Geometry check sheet. Reference: the model listing, model coordinates, mm. A direction names the side the tool comes from. Round coordinates to 2 decimals unless told otherwise and drop trailing zeros. Order: outer loops, then holes, each group sorted by start corner. A loop starts at its lowest first (then second) coordinate and runs counter-clockwise, first axis right, second up. Notation, with made-up numbers: (13.25, 15) -> (26.25, 15) arc R19 ccw to (26.25, 36) -> close; hole circle Ø5 at (51.5, -24). An arc over 180 degrees is marked (long way). Answer as a JSON object with one key per item and string values. Group by question number.
from build123d import *

# Parameters (mm, degrees)
SKETCH2_R           = 2.25
BOSS_EXTRUDE1_DEPTH = 6.35


with BuildPart() as part:
    # Sketch2 → Boss-Extrude1 (new body)
    with BuildSketch(Plane(origin=(0, 0, 71.255), x_dir=(-1, 0, 0), z_dir=(0, 0, -1))):
        with BuildLine():
            Line((-39.5, -8), (39.5, -8))
            ThreePointArc((39.5, -8), (43.035533906, -9.464466094), (44.5, -13))
            Line((44.5, -13), (44.5, -12.496398734))
            ThreePointArc((44.5, -12.496398734), (51.25, -19.246398734), (58, -12.496398734))
            Line((58, -12.496398734), (58, 23.184046239))
            ThreePointArc((58, 23.184046239), (51.25, 29.934046239), (44.5, 23.184046239))
            Line((44.5, 23.184046239), (44.5, 13))
            ThreePointArc((44.5, 13), (43.035533906, 9.464466094), (39.5, 8))
            Line((39.5, 8), (-39.5, 8))
            ThreePointArc((-39.5, 8), (-43.035533906, 9.464466094), (-44.5, 13))
            Line((-44.5, 13), (-44.5, 23.184046239))
            ThreePointArc((-44.5, 23.184046239), (-51.25, 29.934046239), (-58, 23.184046239))
            Line((-58, 23.184046239), (-58, -12.496398734))
            ThreePointArc((-58, -12.496398734), (-51.539037503, -19.240207548), (-44.524753386, -13.073943522))
            Line((-44.524753386, -13.073943522), (-44.481664158, -12.572189046))
            ThreePointArc((-44.481664158, -12.572189046), (-42.880898196, -9.316316058), (-39.5, -8))
        make_face()
        with Locations((47.5, 0)):
            Circle(SKETCH2_R, mode=Mode.SUBTRACT)
        with Locations((-47.5, 0)):
            Circle(SKETCH2_R, mode=Mode.SUBTRACT)
        with Locations((51.25, 23.184046239)):
            Circle(SKETCH2_R, mode=Mode.SUBTRACT)
        with Locations((51.25, -12.496398734)):
            Circle(SKETCH2_R, mode=Mode.SUBTRACT)
        with Locations((-51.25, -12.496398734)):
            Circle(SKETCH2_R, mode=Mode.SUBTRACT)
        with Locations((-51.25, 23.184046239)):
            Circle(SKETCH2_R, mode=Mode.SUBTRACT)
    extrude(amount=BOSS_EXTRUDE1_DEPTH)


solid = part.part
Item 1: Sectioned sample at D-D, the plane x = 51.25. Enter the section's corners in (y, z) (3 decimals), then the cut area to 3 significant figures.
Item 2: Sectioned sample at A-A, the plane y = 0. Enter the section's corners in (x, z) (3 decimals), then the cut area to 3 significant figures.
Item 3: Mould release check, pull along X, two halves, no side actions. Record for faces 1 (the cylindrical face through (53.498, -12.397, 68.124)), 2 (the cylindrical face through (53.498, 23.283, 68.124)), 3 (the flat face through (58, 6, 68)), 4 (the flat face through (1, 0, 64.905)): pulls with the +X half, pulls with the -X half, needs draft (parallel to the pull), parting line crosses it, or undercut.
Item 4: Thickness scan on L1, parallel to Y at x = -51, z = 66.25; L2, parallel to X at y = 18, z = 68; L3, parallel to X at y = 23.5, z = 65.5. Record the ranges inside material, lowest first.
Item 5: Sectioned sample at B-B, the plane y = 19. Enter the section's corners in (x, z) (3 decimals).
Item 6: Set-up check for faces 5 (the flat face through (-44.5, 18, 68)), 6 (the cylindrical face through (42.92, -9.35, 68.12)), 7 (the flat face through (-58, 5, 68)): record each of +Z, -Z, +X, -X, +Y, -Y from which the full face is reachable in a straight line by a thin tool's end or side.
Item 7: Sectioned sample at C-C, the plane z = 67. Enter the section's corners in (x, y).
Item 8: Depth check by flat-ended pin: pin 1 Ø2 at (x, z) = (12.5, 67) entering from -Y. Enter the tip coordinate at first touch or a pass-through.
Result:
{
 "1": {"outline": "(-19.246, 64.905) -> (-14.746, 64.905) -> (-14.746, 71.255) -> (-19.246, 71.255) -> close; (-10.246, 64.905) -> (20.934, 64.905) -> (20.934, 71.255) -> (-10.246, 71.255) -> close; (25.434, 64.905) -> (29.934, 64.905) -> (29.934, 71.255) -> (25.434, 71.255) -> close", "area": "255 mm2"},
 "2": {"outline": "(-58, 64.905) -> (-49.75, 64.905) -> (-49.75, 71.255) -> (-58, 71.255) -> close; (-45.25, 64.905) -> (45.25, 64.905) -> (45.25, 71.255) -> (-45.25, 71.255) -> close; (49.75, 64.905) -> (58, 64.905) -> (58, 71.255) -> (49.75, 71.255) -> close", "area": "679 mm2"},
 "3": {"face 1": "undercut", "face 2": "undercut", "face 3": "pulls with the +X half", "face 4": "needs draft"},
 "4": {"L1": "y = -19.24 to -14.73, -10.26 to 20.95, 25.42 to 29.93", "L2": "x = -58 to -44.5, 44.5 to 58", "L3": "x = -57.99 to -53.48, -49.02 to -44.51, 44.51 to 49.02, 53.48 to 57.99"},
 "5": {"outline": "(-58, 64.905) -> (-44.5, 64.905) -> (-44.5, 71.255) -> (-58, 71.255) -> close; (44.5, 64.905) -> (58, 64.905) -> (58, 71.255) -> (44.5, 71.255) -> close"},
 "6": {"face 5": "+Z, -Z, +Y", "face 6": "+Z, -Z, -Y", "face 7": "+Z, -Z, -X, +Y, -Y"},
 "7": {"outline": "(-58, -12.5) arc R6.75 ccw to (-44.5, -12.5) -> (-44.5, -13) arc R5 cw to (-39.5, -8) -> (39.5, -8) arc R5 cw to (44.48, -12.57) -> (44.52, -13.07) arc R6.75 ccw to (58, -12.5) -> (58, 23.18) arc R6.75 ccw to (44.5, 23.18) -> (44.5, 13) arc R5 cw to (39.5, 8) -> (-39.5, 8) arc R5 cw to (-44.5, 13) -> (-44.5, 23.18) arc R6.75 ccw to (-58, 23.18) -> close; hole circle Ø4.5 at (-51.25, -12.5); hole circle Ø4.5 at (-51.25, 23.18); hole circle Ø4.5 at (-47.5, 0); hole circle Ø4.5 at (47.5, 0); hole circle Ø4.5 at (51.25, -12.5); hole circle Ø4.5 at (51.25, 23.18)"},
 "8": {"pin 1": "stops at y = -8"}
}
